```python
from build123d import *

# Parameters (mm, degrees)
SCHIZZO1_W                   = 2.2
SCHIZZO1_H                   = 2.2
ESTRUSIONE_ESTRUSIONE1_DEPTH = 3.5
SCHIZZO2_R                   = 1.5
ESTRUSIONE_ESTRUSIONE2_DEPTH = 0.5
SCHIZZO3_R                   = 2
ESTRUSIONE_ESTRUSIONE3_DEPTH = 5
SCHIZZO4_R                   = 4
ESTRUSIONE_ESTRUSIONE4_DEPTH = 1
ESTRUSIONE_ESTRUSIONE7_DEPTH = 2
SCHIZZO12_R                  = 1.66147464
ESTRUSIONE_ESTRUSIONE8_DEPTH = 3
SMUSSO4_SIZE                 = 0.2
SMUSSO5_SIZE                 = 0.3


with BuildPart() as part:
    # Schizzo1 → Estrusione-Estrusione1 (new body)
    with BuildSketch(Plane.XY):
        Rectangle(SCHIZZO1_W, SCHIZZO1_H)
    extrude(amount=ESTRUSIONE_ESTRUSIONE1_DEPTH)

    # Schizzo2 → Estrusione-Estrusione2 (add)
    with BuildSketch(Plane.XY.offset(3.5)):
        with Locations(Location((0, 0, 0), (0, 0, 137.166571934))):
            Circle(SCHIZZO2_R)
    extrude(amount=ESTRUSIONE_ESTRUSIONE2_DEPTH)

    # Schizzo3 → Estrusione-Estrusione3 (add)
    with BuildSketch(Plane.XY.offset(4)):
        Circle(SCHIZZO3_R)
    extrude(amount=ESTRUSIONE_ESTRUSIONE3_DEPTH)

    # Schizzo4 → Estrusione-Estrusione4 (add)
    with BuildSketch(Plane.XY.offset(9)):
        Circle(SCHIZZO4_R)
    extrude(amount=ESTRUSIONE_ESTRUSIONE4_DEPTH)

    # Schizzo11 → Estrusione-Estrusione7 (add)
    with BuildSketch(Plane.XY.offset(10)):
        with BuildLine():
            Line((-3.687951879, 2.12924001), (-2.454067959, 8.477022488))
            ThreePointArc((-2.454067959, 8.477022488), (0, 10.5), (2.454067959, 8.477022488))
            Line((2.454067959, 8.477022488), (3.687951879, 2.12924001))
            Line((3.687951879, 2.12924001), (8.568350803, -2.113226049))
            ThreePointArc((8.568350803, -2.113226049), (9.09326674, -5.25), (6.114282844, -6.363796439))
            Line((6.114282844, -6.363796439), (0, -4.25848002))
            Line((0, -4.25848002), (-6.114282844, -6.363796439))
            ThreePointArc((-6.114282844, -6.363796439), (-9.09326674, -5.25), (-8.568350803, -2.113226049))
            Line((-8.568350803, -2.113226049), (-3.687951879, 2.12924001))
        make_face()
    extrude(amount=ESTRUSIONE_ESTRUSIONE7_DEPTH)

    # Schizzo12 → Estrusione-Estrusione8 (add)
    with BuildSketch(Plane.XY.offset(12)):
        with Locations((0, 8)):
            Circle(SCHIZZO12_R)
        with Locations((6.92820323, -4)):
            Circle(SCHIZZO12_R)
        with Locations((-6.92820323, -4)):
            Circle(SCHIZZO12_R)
    extrude(amount=ESTRUSIONE_ESTRUSIONE8_DEPTH)

    # Smusso4
    smusso4_edges = [part.edges().sort_by_distance(p)[0] for p in [
        (-4, 0, 9),
        (-6.128151341, 0.00800698, 10),
        (-9.09326674, -5.25, 10),
        (-3.057141422, -5.31113823, 10),
        (3.057141422, -5.31113823, 10),
        (9.09326674, -5.25, 10),
        (6.128151341, 0.00800698, 10),
        (3.071009919, 5.303131249, 10),
        (0, 10.5, 10),
        (-3.071009919, 5.303131249, 10),
    ]]
    chamfer(smusso4_edges, length=SMUSSO4_SIZE)

    # Smusso5
    smusso5_edges = [part.edges().sort_by_distance(p)[0] for p in [
        (-2, 0, 4),
        (-6.128151341, 0.00800698, 12),
        (-9.09326674, -5.25, 12),
        (-3.057141422, -5.31113823, 12),
        (3.057141422, -5.31113823, 12),
        (9.09326674, -5.25, 12),
        (6.128151341, 0.00800698, 12),
        (3.071009919, 5.303131249, 12),
        (0, 10.5, 12),
        (-3.071009919, 5.303131249, 12),
        (-1.66147464, 8, 15),
        (5.266728591, -4, 15),
        (-8.58967787, -4, 15),
    ]]
    chamfer(smusso5_edges, length=SMUSSO5_SIZE)


solid = part.part
```
For this review, take the finished solid that the model builds, in its own axes (mm). A direction names the side the tool comes from. Give positions to 0.01 mm unless a question says otherwise; leave off trailing zeros. Write each loop counter-clockwise with the first axis right and the second up, starting at its lowest first coordinate (ties: lowest second). Pieces come first, ordered by that corner, then holes. Notation, with made-up numbers: M 14.5,6.5 L 50.5,6.5 A7 ccw 50.5,13.5 Z; hole C 17,51.5 d8. An arc over 180 degrees is marked long. Answer as CSV lines item,"result".
1. Consider section A-A, the plane x = 5. Write out the cut boundary in (y, z), then the cut area to 3 significant figures.
Findings:
outline,"M -5.98,10.2 L -5.77,10 L 0.72,10 L 0.99,10.2 L 0.99,11.7 L 0.59,12 L -5.66,12 L -5.98,11.7 Z"
area,"13.8 mm2"
2. Draft analysis for pull direction X (two halves, no side actions). For faces 1 (the flat face through (3.1, -5.326, 10.939)), 2 (the flat face through (0, 1.1, 2)), 3 (the cylindrical face through (-0.867, -3.905, 9.594)), 4 (the flat face through (-3.08, 5.26, 10.94)), state which applies: +X half, -X half, draft (parallel to the pull), parting line (faces both ways), or undercut.
Findings:
face 1,"undercut"
face 2,"draft"
face 3,"parting line"
face 4,"-X half"
3. For pin 1 (5 mm diameter, centred on x = -1.5, z = 9.5, fed in from -Y); pin 2 (2.5 mm diameter, centred on y = 0, z = 1.5, fed in from +X); pin 3 (2 mm diameter, centred on x = 3, y = -1.5, fed in from -Z), all flat-tipped, find the tip position at first contact; note any pin that passes through.
Findings:
pin 1,"stops at y = -5.6"
pin 2,"stops at x = 1.1"
pin 3,"stops at z = 9"
4. For faces 5 (the cylindrical face through (0, -2, 7)), 6 (the cylindrical face through (8.46, -4.64, 13.33)), 7 (the flat face through (-1.1, 0, 2)), list the 3-axis set-ups (+Z, -Z, +X, -X, +Y, -Y) from which the entire face can be reached by the end or side of a thin tool; tool diameter is ignored.
Findings:
face 5,"-Z"
face 6,"+Z"
face 7,"-Z, -X, +Y, -Y"
5. Wall thickness on line 1 (Z direction, x = -8, y = -4); line 2 (Z direction, x = 0.25, y = 3.5); line 3 (X direction, y = 0, z = 2.5): over which ranges is each line inside the solid? List them lowest first.
Findings:
line 1,"z = 10 to 15"
line 2,"z = 9 to 12"
line 3,"x = -1.1 to 1.1"
6. Consider section C-C, the plane y = 0. Write out the cut boundary in (x, z), then the cut area to 3 significant figures.
Findings:
outline,"M -6.14,10.2 L -5.83,10 L -4,10 L -4,9.2 L -3.8,9 L -2,9 L -2,4.3 L -1.7,4 L -1.5,4 L -1.5,3.5 L -1.1,3.5 L -1.1,0 L 1.1,0 L 1.1,3.5 L 1.5,3.5 L 1.5,4 L 1.7,4 L 2,4.3 L 2,9 L 3.8,9 L 4,9.2 L 4,10 L 5.83,10 L 6.14,10.2 L 6.14,11.7 L 5.68,12 L -5.68,12 L -6.14,11.7 Z"
area,"61.4 mm2"
7. Consider section D-D, the plane z = 2.5. Write out the cut boundary in (x, y).
Findings:
outline,"M -1.1,-1.1 L 1.1,-1.1 L 1.1,1.1 L -1.1,1.1 Z"
8. Consider section B-B, the plane z = 7.75. Write out the cut boundary in (x, y).
Findings:
outline,"C 0,0 d4"
